Geometry: see drawing. Coordinates: mm, zero at the bounding-box minimum. A direction names the side the tool comes from. Coordinates: 2 decimals unless noted, no trailing zeros. Order: outer loops, then holes, each group sorted by start corner. A loop starts at its lowest first (then second) coordinate and runs counter-clockwise, first axis right, second up. Notation, with made-up numbers: M 37.25,-36 L 86.25,-36 A16 cw 86.25,-20 Z; hole C 54,66 d5. An arc over 180 degrees is marked long. Answer in a Markdown table with one row per item.
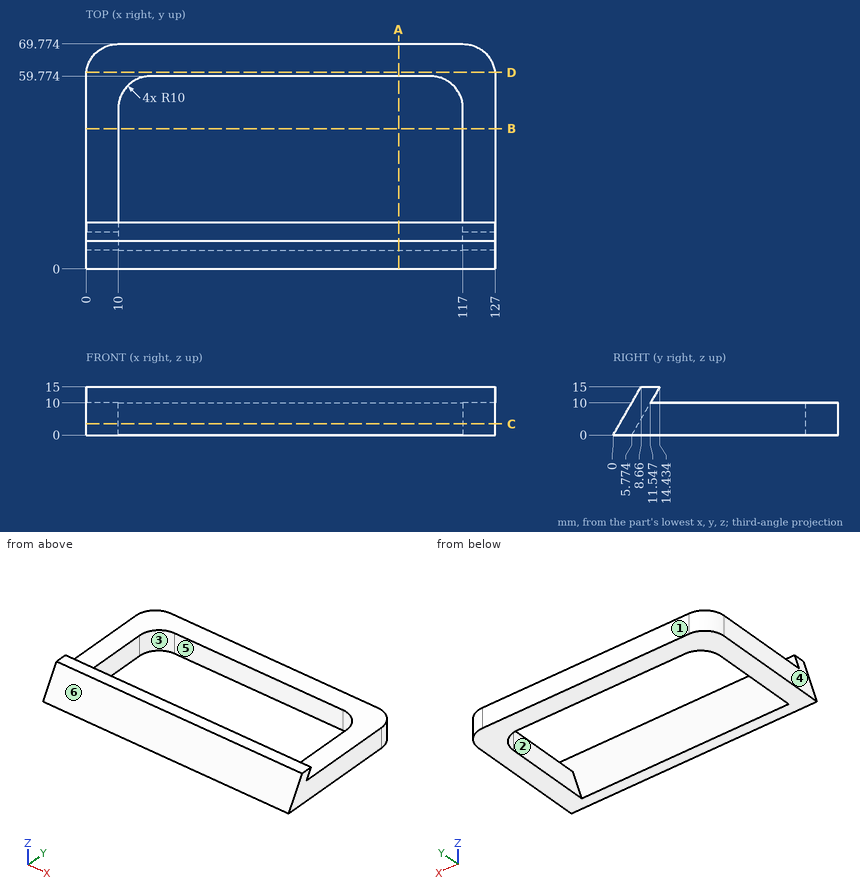
1) Material intervals for probe 1 along X at (y, z) = (31.5, 1.25); probe 2 along Y at (x, z) = (22, 5.75) (1 decimal); probe 3 along Y at (x, z) = (95, 2) (1 decimal), sorted ascending.
Resolved:
| item | result |
|---|---|
| probe 1 | x = 0 to 10, 117 to 127 |
| probe 2 | y = 3.3 to 9.1, 59.8 to 69.8 |
| probe 3 | y = 1.2 to 6.9, 59.8 to 69.8 |
2) Cut plane B-B, the plane y = 43.5. Output: boundary loops of the cut face in (x, z), and give its area (3 significant figures).
Resolved:
| item | result |
|---|---|
| outline | M 0,0 L 10,0 L 10,10 L 0,10 Z; M 117,0 L 127,0 L 127,10 L 117,10 Z |
| area | 200 mm2 |
3) Contact query for flat-ended pins moving along their axis: pin 1 (12 mm diameter, centred on x = 89, y = 53.5, fed in from +Z); pin 2 (5 mm diameter, centred on x = 99.5, z = 10, fed in from -Y); pin 3 (5 mm diameter, centred on x = 88, z = 9.5, fed in from -Y); pin 4 (3 mm diameter, centred on x = 57.5, z = 5, fed in from -Y). Output: stop coordinate, or through.
Resolved:
| item | result |
|---|---|
| pin 1 | passes through |
| pin 2 | stops at y = 4.33 |
| pin 3 | stops at y = 4.04 |
| pin 4 | stops at y = 2.02 |
4) Cut plane A-A, the plane x = 97. Output: boundary loops of the cut face in (y, z), and give its area (3 significant figures).
Resolved:
| item | result |
|---|---|
| outline | M 0,0 L 5.77,0 L 14.43,15 L 8.66,15 Z; M 59.77,0 L 69.77,0 L 69.77,10 L 59.77,10 Z |
| area | 187 mm2 |
5) Mould query, pull axis X, two halves, no side actions, for the marked faces 4, 5 and 6. Classes: +X half, -X half, draft (parallel to the pull), parting line (faces both ways), or undercut.
Resolved:
| item | result |
|---|---|
| face 4 | -X half |
| face 5 | undercut |
| face 6 | draft |
6) Cut plane C-C, the plane z = 3.5. Output: boundary loops of the cut face in (x, y) (1 decimal), and give its area (3 significant figures).
Resolved:
| item | result |
|---|---|
| outline | M 0,2 L 127,2 L 127,59.8 A10 ccw 117,69.8 L 10,69.8 A10 ccw 0,59.8 Z; hole M 10,7.8 L 117,7.8 L 117,49.8 A10 ccw 107,59.8 L 20,59.8 A10 ccw 10,49.8 Z |
| area | 3,040 mm2 |
7) Reachability of the marked faces 1, 2 and 3 from +Z, -Z, +X, -X, +Y, -Y: full face, straight path, thin tool, end or side. Return the list, or none.
Resolved:
| item | result |
|---|---|
| face 1 | +Z, -Z, +X, -X, +Y |
| face 2 | -Z |
| face 3 | +Z, -Z |
8) Cut plane D-D, the plane y = 61. Output: boundary loops of the cut face in (x, z) (1 decimal).
Resolved:
| item | result |
|---|---|
| outline | M 0.1,0 L 126.9,0 L 126.9,10 L 0.1,10 Z |
